Check sheet for the modelled part. Datum: model origin and axes. Units: mm. Face numbers are marked on the shaded views. Coordinates: 2 decimals unless noted, no trailing zeros. Loops run counter-clockwise (first coordinate to the right, second up) from the corner with the lowest first, then second, coordinate; pieces in that order, holes last. Notation, with made-up numbers: M 35,86 L 43,86 A14 ccw 43,105 Z; hole C -34.75,56.5 d1. An arc over 180 degrees is marked long. Use CSV: the item, a comma, the result in double quotes. Start each with the question number.
(1) Section check A-A on y = 395. Record the cut outline in (x, z).
(2) Go/stop test with a flat-tipped pin: pin 1 Ø3 at (x, z) = (-11.5, 93) entering from -Y. Record where the tip stops, or that it passes through.
(3) Draft check along Z on the marked faces 1, 2 and 3. Enter one of: pulls with the +Z half, pulls with the -Z half, needs draft (parallel to the pull), parting line crosses it, or undercut.
(4) Section check B-B on z = 105. Record the cut outline in (x, y).
(5) Scan lines: line 1 (Y direction, x = -8.25, z = 90); line 2 (Y direction, x = -3.75, z = 58.5); line 3 (Y direction, x = -1, z = 26.5). Record each from-to range of solid material in increasing order.
(6) Section check C-C on x = -14. Give the number of separate pieces and of enclosed holes in the cut face, and give its area (3 significant figures).
from build123d import *

# Parameters (mm, degrees)
SKETCH_2_W                  = 20
SKETCH_2_H                  = 500
SM_BASE_FLANGE_1_DEPTH      = 120
SKETCH_3_R                  = 28
CUT_EXTRUDE_1_DEPTH         = 515.587213211
CUT_EXTRUDE_START           = -20
CUT_EXTRUDE_2_DEPTH         = 20
HOLE_WIZARD_14_0_14_1_D     = 14
HOLE_WIZARD_14_0_14_1_DEPTH = 45
HOLE_WIZARD_14_0_14_1_TIP   = 4.206024333


# Read off the part's stored shape, not the designer's step: 切除-拉伸2
# Sheet-metal steps are written as plain solids
with BuildPart() as part:
    # 草图2 → 基体-法兰1 (new body)
    with BuildSketch(Plane.XY):
        with Locations((-10, 250)):
            Rectangle(SKETCH_2_W, SKETCH_2_H)
    extrude(amount=SM_BASE_FLANGE_1_DEPTH)

    # 草图3 → 切除-拉伸1 (cut, through all)
    with BuildSketch(Plane(origin=(0, 0, 0), x_dir=(0, 0, -1), z_dir=(1, 0, 0))):
        with Locations(Location((-60, 60, 0), (0, 0, 90))):
            Circle(SKETCH_3_R)
        with Locations(Location((-60, 440, 0), (0, 0, 90))):
            Circle(SKETCH_3_R)
    extrude(amount=-CUT_EXTRUDE_1_DEPTH, mode=Mode.SUBTRACT)

    # 切除-拉伸2 outline → 切除-拉伸2 (cut)
    with BuildSketch(Plane.ZY.offset(20).offset(CUT_EXTRUDE_START)):
        with BuildLine():
            ThreePointArc((60, 0), (17.573593129, 17.573593129), (0, 60))
            Line((0, 60), (0, 0))
            Line((0, 0), (60, 0))
        make_face()
        with BuildLine():
            ThreePointArc((120, 60), (102.426406871, 17.573593129), (60, 0))
            Line((60, 0), (120, 0))
            Line((120, 0), (120, 60))
        make_face()
        with BuildLine():
            Line((0, 500), (0, 440))
            ThreePointArc((0, 440), (17.573593129, 482.426406871), (60, 500))
            Line((60, 500), (0, 500))
        make_face()
        with BuildLine():
            Line((120, 500), (60, 500))
            ThreePointArc((60, 500), (102.426406871, 482.426406871), (120, 440))
            Line((120, 440), (120, 500))
        make_face()
    extrude(amount=CUT_EXTRUDE_2_DEPTH, mode=Mode.SUBTRACT)

    # Ø14.0 (14) 直径孔1
    with Locations(Plane(origin=(0, 0, 0), x_dir=(0, 0, -1), z_dir=(1, 0, 0))):
        with Locations((-60, 485), (-105, 440), (-60, 395), (-15, 440), (-90, 225.486069721), (-90, 285.486069721), (-30, 285.486069721), (-30, 225.486069721), (-30, 345.486069721), (-90, 345.486069721)):
            Hole(HOLE_WIZARD_14_0_14_1_D / 2, depth=HOLE_WIZARD_14_0_14_1_DEPTH)
            with Locations((0, 0, -(HOLE_WIZARD_14_0_14_1_DEPTH + HOLE_WIZARD_14_0_14_1_TIP / 2))):  # 118° drill point
                Cone(0, HOLE_WIZARD_14_0_14_1_D / 2, HOLE_WIZARD_14_0_14_1_TIP, mode=Mode.SUBTRACT)


solid = part.part
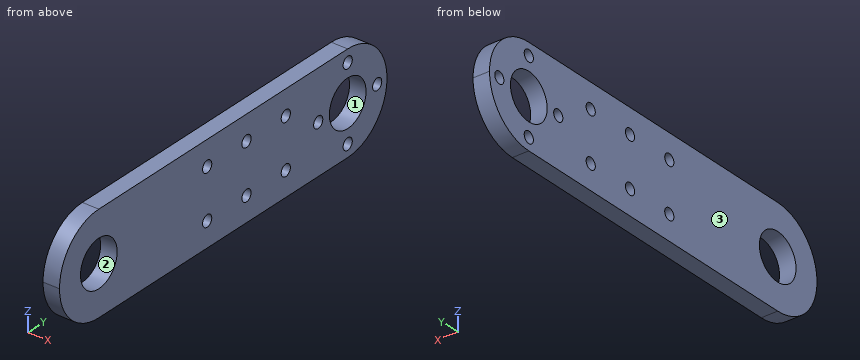
Outcome:
1,outline,"M -20,0 L 0,0 L 0,53 L -20,53 Z; M -20,67 L 0,67 L 0,120 L -20,120 Z"
2,pin 1,"stops at y = 8.93"
3,face 1,"undercut"
3,face 2,"undercut"
3,face 3,"needs draft"
4,outline,"M -20,20.31 L 0,20.31 L 0,433 L -20,433 Z; M -20,447 L 0,447 L 0,479.69 L -20,479.69 Z"
5,line 1,"y = 8.04 to 218.49, 232.49 to 278.49, 292.49 to 338.49, 352.49 to 491.96"
5,line 2,"y = 0.02 to 32.04, 87.96 to 388.16, 401.84 to 412.04, 467.96 to 478.16, 491.84 to 499.98"
5,line 3,"y = 10.22 to 219.42, 231.55 to 279.42, 291.55 to 339.42, 351.55 to 489.78"
6,separate pieces,"1"
6,enclosed holes,"12"
6,area,"50,400 mm²"
